from build123d import *

# Parameters (mm, degrees)
PAD001_DEPTH = 50
PAD_DEPTH    = 50


with BuildPart() as obj1:
    # Sketch → Pad001 (new body)
    with BuildSketch(Plane.YZ):
        with BuildLine():
            Line((-7, 0), (109.440979, 10))
            ThreePointArc((130.889931, 4.362511), (120.653215, 9.037037), (109.440979, 10))
            ThreePointArc((130.889931, 4.362511), (137.615463, 1.115515), (145, 0))
            ThreePointArc((145, 0), (152.631281, 1.193204), (159.534108, 4.658916))
            Line((159.534108, 4.658916), (195, 30))
            Line((195, 30), (195, 36))
            Line((159.534108, 10.658916), (195, 36))
            ThreePointArc((145, 6), (152.631281, 7.193204), (159.534108, 10.658916))
            ThreePointArc((130.889584, 10.362749), (137.615262, 7.115577), (145, 6))
            ThreePointArc((130.889584, 10.362749), (120.652594, 15.03754), (109.44, 16.000536))
            Line((-7, 6), (109.44, 16.000536))
            Line((-7, 6), (-7, 0))
        make_face()
    extrude(amount=PAD001_DEPTH)


with BuildPart() as obj1_1:
    # Body001 placement: moved
    add(obj1.part.moved(Location((-25, 0, 0))))


with BuildPart() as common:
    # Sketch003 → Pad (new body)
    with BuildSketch(Plane.XY):
        with BuildLine():
            Line((18, 190.020199), (18, 140.020199))
            ThreePointArc((17.359364, 138.714947), (17.831207, 139.293202), (18, 140.020199))
            Line((17.359364, 138.714947), (16.151931, 137.781227))
            ThreePointArc((16.151931, 137.781227), (8.907519, 128.823515), (6.449131, 117.568362))
            Line((6.449131, 117.568362), (8.498705, 0.148345))
            ThreePointArc((0, -8.5), (6.062629, -5.957729), (8.498705, 0.148345))
            ThreePointArc((-8.498705, 0.148345), (-6.062629, -5.957729), (0, -8.5))
            Line((-6.449131, 117.568362), (-8.498705, 0.148345))
            ThreePointArc((-6.449131, 117.568362), (-8.907519, 128.823515), (-16.151931, 137.781227))
            Line((-17.359364, 138.714947), (-16.151931, 137.781227))
            ThreePointArc((-18, 140.020199), (-17.831207, 139.293202), (-17.359364, 138.714947))
            Line((-18, 190.020199), (-18, 140.020199))
            ThreePointArc((-14.009771, 190.217657), (-16.098849, 192.017755), (-18, 190.020199))
            Line((-14.009771, 190.217657), (-10.040229, 150.207506))
            ThreePointArc((-10.040229, 150.207506), (-8.052525, 148.404965), (-6.060276, 150.202482))
            Line((-6.060276, 150.202482), (-1.989724, 190.202482))
            ThreePointArc((0, 192), (-1.340716, 191.484076), (-1.989724, 190.202482))
            ThreePointArc((1.989724, 190.202482), (1.340716, 191.484076), (0, 192))
            Line((6.060276, 150.202482), (1.989724, 190.202482))
            ThreePointArc((6.060276, 150.202482), (8.052525, 148.404965), (10.040229, 150.207506))
            Line((14.009771, 190.217657), (10.040229, 150.207506))
            ThreePointArc((18, 190.020199), (16.098849, 192.017755), (14.009771, 190.217657))
        make_face()
    extrude(amount=PAD_DEPTH)


with BuildPart() as common_1:
    # Body placement: moved
    add(common.part.moved(Location((0, 0, -8))))

    # Common: intersect obj1
    add(obj1_1.part, mode=Mode.INTERSECT)


solid = common_1.part
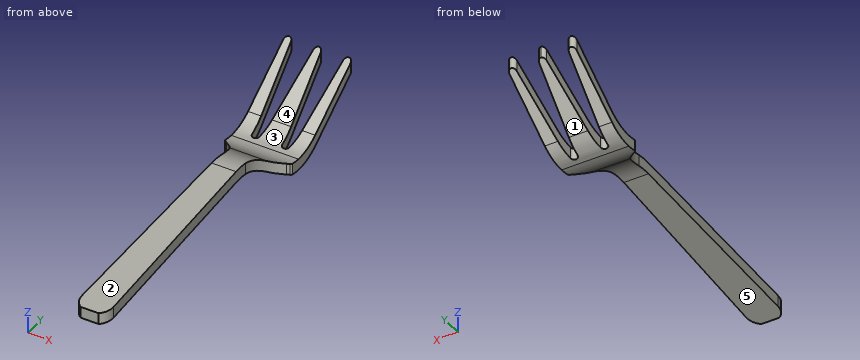
Part model, mm, in its own coordinate system. Face numbers are marked on the shaded views. A direction names the side the tool comes from. Give positions to 0.01 mm unless a question says otherwise; leave off trailing zeros. Loops run counter-clockwise (first coordinate to the right, second up) from the corner with the lowest first, then second, coordinate; pieces in that order, holes last. Notation, with made-up numbers: (86, -7) -> (108, -7) arc R18 cw to (108, 5) -> close; hole circle Ø2 at (35, 29.5). An arc over 180 degrees is marked (long way). Write each question's results on one line, items separated by ' | '. Start each with the question number.
Q1. Band-saw the part on A-A on z = 23. List the corners of the cut face in (x, y), plus the area to 3 significant figures.
Q2. Pull direction Y, two halves, no side cores. Call the marked faces 1, 2 and 3: +Y half, -Y half, draft (parallel to the pull), parting line (faces both ways), or undercut.
Q3. Band-saw the part on C-C on y = 107. List the corners of the cut face in (x, z), plus the area to 3 significant figures.
Q4. Pin check, flat tips, straight feed: P1, Ø6, axis at x = 8.5, y = 65, coming from the -Z side; P2, Ø1, axis at x = 12.5, z = 15, coming from the -Y side; P3, Ø12, axis at x = 7.5, z = 28.5, coming from the -Y side. Stop position of each tip, or through.
Q5. Band-saw the part on B-B on y = 78.5. List the corners of the cut face in (x, z).
Q6. Which spindle directions (+Z, -Z, +X, -X, +Y, -Y) get a long thin tool onto all of the face, cutting with end or side? Do the marked faces 4 and 5. Say none if no direction does.
Q7. Wall check: L1, parallel to X at y = 164, z = 10; L2, parallel to Z at x = 3.5, y = 5; L3, parallel to Z at x = 0.5, y = 145. Give the ranges that are in metal, low to high.
Results are:
1) outline: (-18, 176.81) -> (-12.68, 176.81) -> (-13.51, 185.2) -> (-18, 185.2) -> close; (-3.35, 176.81) -> (3.35, 176.81) -> (2.5, 185.2) -> (-2.5, 185.2) -> close; (12.68, 176.81) -> (18, 176.81) -> (18, 185.2) -> (13.51, 185.2) -> close | area: 132 mm²
2) face 1: +Y half | face 2: -Y half | face 3: undercut
3) outline: (-6.63, 9.79) -> (6.63, 9.79) -> (6.63, 15.79) -> (-6.63, 15.79) -> close | area: 79.6 mm²
4) P1: stops at z = 5.94 | P2: stops at y = 164.91 | P3: stops at y = 178.71
5) outline: (-7.13, 7.34) -> (7.13, 7.34) -> (7.13, 13.34) -> (-7.13, 13.34) -> close
6) face 4: +Z, +X, -X | face 5: -Z, +X, -X
7) L1: x = -18 to -11.41, -4.66 to 4.66, 11.41 to 18 | L2: z = 1.03 to 7.03 | L3: z = 0 to 6
